Check sheet for the drawn part. Datum: minimum x, y, z corner. Units: mm. A direction names the side the tool comes from. Give positions to 0.01 mm unless a question says otherwise; leave off trailing zeros. Order: outer loops, then holes, each group sorted by start corner. A loop starts at its lowest first (then second) coordinate and runs counter-clockwise, first axis right, second up.
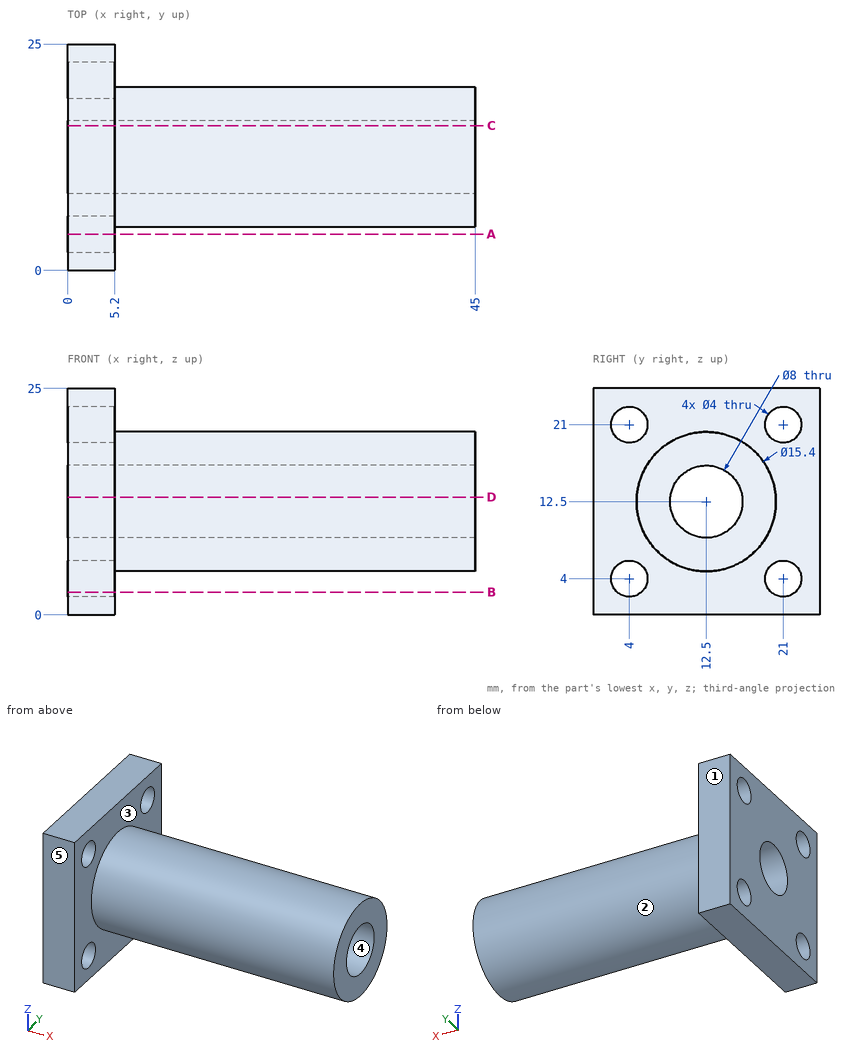
(1) Set-up check for the marked faces 1 and 2: record each of +Z, -Z, +X, -X, +Y, -Y from which the full face is reachable in a straight line by a thin tool's end or side.
Solved:
face 1: +Z, -Z, +X, -X, +Y
face 2: +X
(2) Go/stop test with flat-tipped pins: pin 1 (2 mm diameter, centred on x = 7.5, z = 9.5, fed in from +Y); pin 2 (3.5 mm diameter, centred on y = 4, z = 4, fed in from +X); pin 3 (4 mm diameter, centred on x = 28, z = 21, fed in from +Y); pin 4 (2 mm diameter, centred on x = 31, y = 18.5, fed in from +Z). Record where each tip stops, or that it passes through.
Solved:
pin 1: stops at y = 19.94
pin 2: passes through
pin 3: stops at y = 16.63
pin 4: stops at z = 18.36
(3) Release check for a two-part mould opening along Y. For the marked faces 3, 4 and 5 record: pulls with the +Y half, pulls with the -Y half, needs draft (parallel to the pull), parting line crosses it, or undercut.
Solved:
face 3: needs draft
face 4: undercut
face 5: pulls with the -Y half
(4) Section check C-C, the plane y = 16. Enter the section's corners in (x, z), then the cut area to 3 significant figures.
Solved:
outline: (0, 0) - (5.2, 0) - (5.2, 5.64) - (45, 5.64) - (45, 10.56) - (0, 10.56) - close; (0, 14.44) - (45, 14.44) - (45, 19.36) - (5.2, 19.36) - (5.2, 25) - (0, 25) - close
area: 502 mm2
(5) Section check B-B, the plane z = 2.5. Enter the section's corners in (x, y).
Solved:
outline: (0, 0) - (5.2, 0) - (5.2, 2.68) - (0, 2.68) - close; (0, 5.32) - (5.2, 5.32) - (5.2, 19.68) - (0, 19.68) - close; (0, 22.32) - (5.2, 22.32) - (5.2, 25) - (0, 25) - close
(6) Scan lines: line 1 (Z direction, x = 2.75, y = 4); line 2 (Z direction, x = 27, y = 12.5); line 3 (X direction, y = 2.25, z = 13). Record each from-to range of solid material in increasing order.
Solved:
line 1: z = 0 to 2, 6 to 19, 23 to 25
line 2: z = 4.8 to 8.5, 16.5 to 20.2
line 3: x = 0 to 5.2
(7) Section check D-D, the plane z = 13. Enter the section's corners in (x, y), then the cut area to 3 significant figures.
Solved:
outline: (0, 0) - (5.2, 0) - (5.2, 4.82) - (45, 4.82) - (45, 8.53) - (0, 8.53) - close; (0, 16.47) - (45, 16.47) - (45, 20.18) - (5.2, 20.18) - (5.2, 25) - (0, 25) - close
area: 384 mm2
(8) Section check A-A, the plane y = 4. Enter the section's corners in (x, z).
Solved:
outline: (0, 0) - (5.2, 0) - (5.2, 2) - (0, 2) - close; (0, 6) - (5.2, 6) - (5.2, 19) - (0, 19) - close; (0, 23) - (5.2, 23) - (5.2, 25) - (0, 25) - close
